from build123d import *

# Parameters (mm, degrees)
BOSS_EXTRUDE1_DEPTH = 450
CUT_EXTRUDE1_DEPTH  = 451.888012704


with BuildPart() as part:
    # Sketch1 → Boss-Extrude1 (new body)
    with BuildSketch(Plane(origin=(0, 0, 0), x_dir=(0, 0, -1), z_dir=(1, 0, 0))):
        Polygon((0, 0), (20, 0), (20, 3.461178467), (3.461178467, 3.461178467), (3.461178467, 20), (0, 20), align=None)
    extrude(amount=BOSS_EXTRUDE1_DEPTH)

    # Sketch2 → Cut-Extrude1 (cut, through all)
    with BuildSketch(Plane(origin=(0, 0, 0), x_dir=(1, 0, 0), z_dir=(0, 0, -1))):
        Polygon((0, -20), (0, 0), (20, -20), align=None)
    extrude(amount=CUT_EXTRUDE1_DEPTH, mode=Mode.SUBTRACT)


solid = part.part
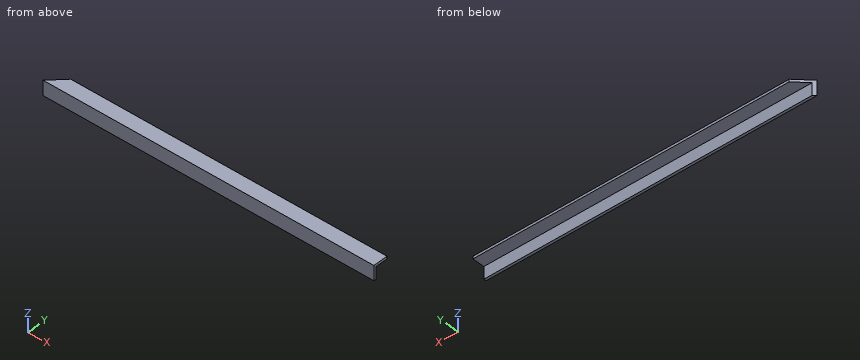
Here's how the part is built. I have some questions about the finished solid (model axes, mm). Coordinates: 2 decimals unless noted, no trailing zeros. Write each loop counter-clockwise with the first axis right and the second up, starting at its lowest first coordinate (ties: lowest second). Pieces come first, ordered by that corner, then holes.
Item 1: If I drill on line 1 (Y direction, x = 45, z = -19); line 2 (Z direction, x = 234.5, y = 14); line 3 (X direction, y = 18.75, z = -3), over which ranges is the centre line in solid material (lowest first)?
Item 2: I want a section at C-C on y = 12. Write out the boundary of the cut face in (x, z), and give its area (3 significant figures).
Item 3: Will these pins go through, and if not, where does the flat tip stop? pin 1 (5 mm diameter, centred on x = 285, y = 13.5, fed in from -Z); pin 2 (2 mm diameter, centred on x = 172, y = 7.5, fed in from +Z); pin 3 (3 mm diameter, centred on x = 72, z = -13.5, fed in from +Y).
Item 4: I want a section at A-A on x = 33.5. Write out the boundary of the cut face in (y, z).
Item 5: I want a section at B-B on z = -8. Write out the boundary of the cut face in (x, y), and give its area (3 significant figures).
Findings below:
1. line 1: y = 0 to 3.46
1. line 2: z = -3.46 to 0
1. line 3: x = 18.75 to 450
2. outline: (12, -3.46) - (450, -3.46) - (450, 0) - (12, 0) - close
2. area: 1,520 mm2
3. pin 1: stops at z = -3.46
3. pin 2: stops at z = 0
3. pin 3: stops at y = 3.46
4. outline: (0, -20) - (3.46, -20) - (3.46, -3.46) - (20, -3.46) - (20, 0) - (0, 0) - close
5. outline: (0, 0) - (450, 0) - (450, 3.46) - (3.46, 3.46) - close
5. area: 1,550 mm2
